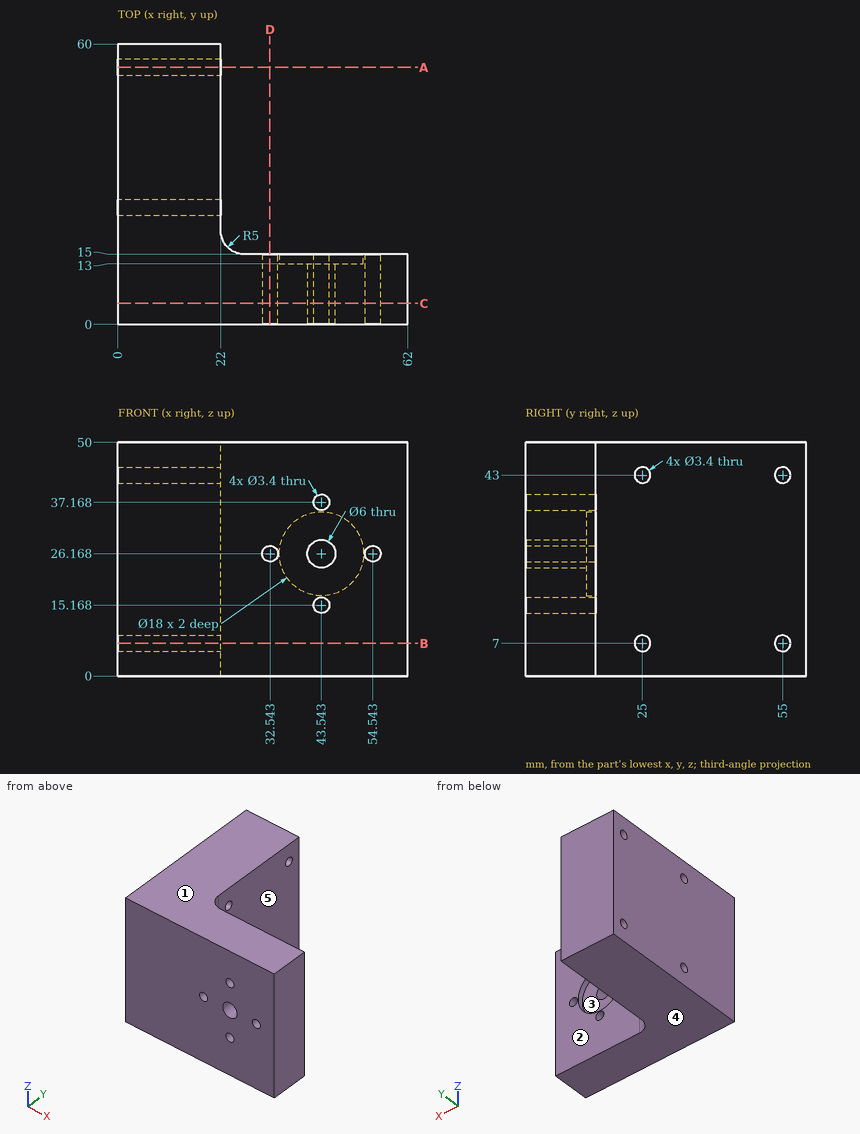
Source: three-view drawing plus pictorial views. Frame: mm from the lowest corner of the part. A direction names the side the tool comes from. Round coordinates to 2 decimals unless told otherwise and drop trailing zeros. Loops run counter-clockwise (first coordinate to the right, second up) from the corner with the lowest first, then second, coordinate; pieces in that order, holes last. Notation, with made-up numbers: M 41,36 L 86,36 A12 cw 86,59 Z; hole C 87,76.5 d5. An arc over 180 degrees is marked long. Put each result on its own line as item: value. Start each with the question number.
(1) Contact query for flat-ended pins moving along their axis: pin 1 Ø5 at (y, z) = (29.5, 30) entering from +X; pin 2 Ø5.5 at (x, z) = (32.54, 26.17) entering from +Y; pin 3 Ø10.5 at (x, z) = (43.5, 27.5) entering from +Y. Output: stop coordinate, or through.
(2) Set-up query: the marked faces 1 and 2. Return all of +Z, -Z, +X, -X, +Y, -Y with unobstructed straight access to the full face (end or side cutting, diameter ignored); none if empty.
(3) Material intervals for line 1 along X through (y, z) = (57.5, 35); line 2 along Y through (x, z) = (32.5, 17.5); line 3 along Y through (x, z) = (46.5, 32.5), sorted ascending. Write a range as [from, to].
(4) Section query D-D (x = 32.5). Return loops of the section in (y, z), then the cut area to 3 significant figures.
(5) Section query A-A (y = 55). Return loops of the section in (x, z).
(6) Section query C-C (y = 4.5). Return loops of the section in (x, z).
(7) Section query B-B (z = 7). Return loops of the section in (x, y), then the cut area to 3 significant figures.
(8) Draft query along Z for the marked faces 3, 4 and 5. Return one class per face: +Z half, -Z half, draft (parallel to the pull), parting line (faces both ways), or undercut.
Findings below:
1. pin 1: stops at x = 22
1. pin 2: stops at y = 15
1. pin 3: stops at y = 13
2. face 1: +Z, +X, -X, +Y, -Y
2. face 2: +Z, -Z, +X, +Y
3. line 1: x = [0, 22]
3. line 2: y = [0, 15]
3. line 3: y = [0, 13]
4. outline: M 0,0 L 15,0 L 15,24.47 L 0,24.47 Z; M 0,27.87 L 15,27.87 L 15,50 L 0,50 Z
4. area: 699 mm2
5. outline: M 0,0 L 22,0 L 22,5.3 L 0,5.3 Z; M 0,8.7 L 22,8.7 L 22,41.3 L 0,41.3 Z; M 0,44.7 L 22,44.7 L 22,50 L 0,50 Z
6. outline: M 0,0 L 62,0 L 62,50 L 0,50 Z; hole C 32.54,26.17 d3.4; hole C 43.54,26.17 d6; hole C 43.54,15.17 d3.4; hole C 43.54,37.17 d3.4; hole C 54.54,26.17 d3.4
7. outline: M 0,0 L 62,0 L 62,15 L 27,15 A5 cw 22,20 L 22,23.3 L 0,23.3 Z; M 0,26.7 L 22,26.7 L 22,53.3 L 0,53.3 Z; M 0,56.7 L 22,56.7 L 22,60 L 0,60 Z
7. area: 1,780 mm2
8. face 3: undercut
8. face 4: -Z half
8. face 5: draft
